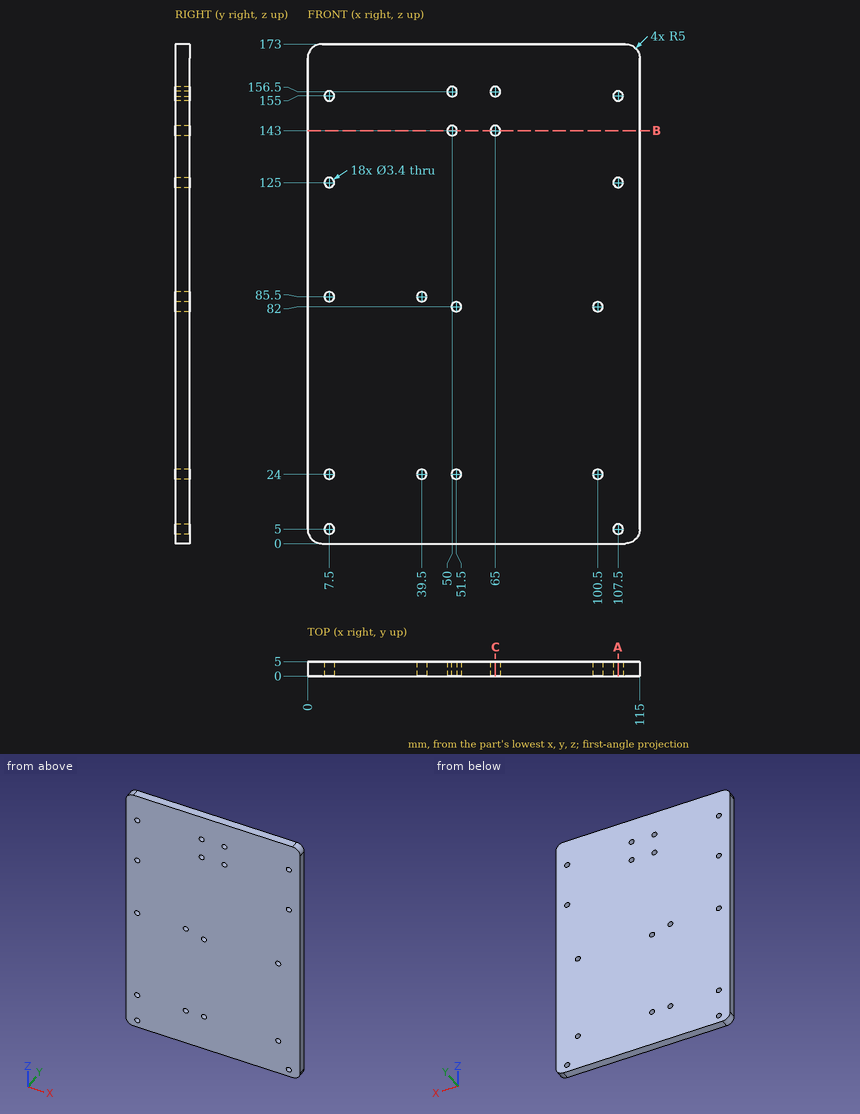
Can you work these out from the drawing? Everything is in mm from the part's minimum corner. Give positions to 0.01 mm unless a question says otherwise; leave off trailing zeros. Loops run counter-clockwise (first coordinate to the right, second up) from the corner with the lowest first, then second, coordinate; pieces in that order, holes last. Notation, with made-up numbers: (56, -32) -> (72, -32) arc R18 ccw to (72, -4) -> close; hole circle Ø6 at (23, 3). An arc over 180 degrees is marked (long way). Return JSON: item names as keys, results as strings.
Item 1: I need wall thicknesses on L1, parallel to Z at x = 7.5, y = 3.6; L2, parallel to Z at x = 65, y = 3.95; L3, parallel to Z at x = 50, y = 3.8. Which ranges of each line are inside material? Lowest first, please. Write a range as from..to.
Geometry results:
{"L1": "z = 0..3.3, 6.7..22.3, 25.7..83.8, 87.2..123.3, 126.7..153.3, 156.7..173", "L2": "z = 0..141.3, 144.7..154.8, 158.2..173", "L3": "z = 0..23.2, 24.8..81.2, 82.8..141.3, 144.7..154.8, 158.2..173"}
Item 2: If we section it at A-A on x = 107.5: List the corners of the cut face in (y, z) for me, plus the area to 3 significant figures.
Geometry results:
{"outline": "(0, 0) -> (5, 0) -> (5, 3.3) -> (0, 3.3) -> close; (0, 6.7) -> (5, 6.7) -> (5, 123.3) -> (0, 123.3) -> close; (0, 126.7) -> (5, 126.7) -> (5, 153.3) -> (0, 153.3) -> close; (0, 156.7) -> (5, 156.7) -> (5, 173) -> (0, 173) -> close", "area": "814 mm²"}
Item 3: If we section it at B-B on z = 143: List the corners of the cut face in (x, y) for me, plus the area to 3 significant figures.
Geometry results:
{"outline": "(0, 0) -> (48.3, 0) -> (48.3, 5) -> (0, 5) -> close; (51.7, 0) -> (63.3, 0) -> (63.3, 5) -> (51.7, 5) -> close; (66.7, 0) -> (115, 0) -> (115, 5) -> (66.7, 5) -> close", "area": "541 mm²"}
Item 4: If we section it at C-C on x = 65: List the corners of the cut face in (y, z) for me, plus the area to 3 significant figures.
Geometry results:
{"outline": "(0, 0) -> (5, 0) -> (5, 141.3) -> (0, 141.3) -> close; (0, 144.7) -> (5, 144.7) -> (5, 154.8) -> (0, 154.8) -> close; (0, 158.2) -> (5, 158.2) -> (5, 173) -> (0, 173) -> close", "area": "831 mm²"}
